from build123d import *

# Parameters (mm, degrees)
CHAMFER_1_SIZE           = 1
SKETCH_4_W               = 2
SKETCH_4_H               = 1
CUT_EXTRUDE_1_DEPTH      = 35.092374778
CUT_EXTRUDE_2_REACH      = 36.092
PATTERN_CIRCULAR_3_COUNT = 18
SKETCH_7_R               = 25
CUT_EXTRUDE_3_DEPTH      = 21
SKETCH_8_R               = 5
EXTRUDE_1_DEPTH          = 7
SKETCH_10_R              = 3
CUT_EXTRUDE_4_DEPTH      = 10
SKETCH_11_R              = 1.525
CUT_EXTRUDE_5_DEPTH      = 46


with BuildPart() as part:
    # 草图1 → 旋转1 (revolve)
    with BuildSketch(Plane.XY, mode=Mode.PRIVATE) as revolve_1_sk:
        Polygon((0, 2.7506), (0, 13.753), (28, 13.753), (28, 5.5012), (20, 5.5012), (20, 2.7506), align=None)
    revolve(revolve_1_sk.sketch.rotate(Axis((0, 0, 0), (1, 0, 0)), 90), axis=Axis((0, 0, 0), (1, 0, 0)))

    # 倒角1
    chamfer_1_edges = [part.edges().sort_by_distance(p)[0] for p in [
        (20, 0, -2.7506),
        (0, 0, -2.7506),
    ]]
    chamfer(chamfer_1_edges, length=CHAMFER_1_SIZE)

    # 草图4 → 切除-拉伸1 (cut, through all)
    with BuildSketch(Plane.ZY):
        with Locations((0, 3.062381775)):
            Rectangle(SKETCH_4_W, SKETCH_4_H)
    extrude(amount=-CUT_EXTRUDE_1_DEPTH, mode=Mode.SUBTRACT)

    # 草图6 → 切除-拉伸2 (cut, up to next)
    with BuildSketch(Plane(origin=(0, 0, 0), x_dir=(0, 0, -1), z_dir=(1, 0, 0)), mode=Mode.PRIVATE) as cut_extrude_2_sk1:
        with BuildLine():
            Line((1.574067282, 13.17215513), (1.548371997, 12.962883824))
            ThreePointArc((1.548371997, 12.962883824), (0, 11.593), (-1.548371997, 12.962883824))
            Line((-1.548371997, 12.962883824), (-1.574067282, 13.17215513))
            ThreePointArc((-1.574067282, 13.17215513), (-1.761240253, 13.496717776), (-2.124642597, 13.587895453))
            ThreePointArc((-2.124642597, 13.587895453), (-2.36143787, 13.548749765), (-2.597513963, 13.505477785))
            Line((-2.597513963, 13.505477785), (-2.794161951, 15.107047128))
            ThreePointArc((-2.794161951, 15.107047128), (0, 15.363274844), (2.794161951, 15.107047128))
            Line((2.794161951, 15.107047128), (2.597513963, 13.505477785))
            ThreePointArc((2.597513963, 13.505477785), (2.36143787, 13.548749765), (2.124642597, 13.587895453))
            ThreePointArc((2.124642597, 13.587895453), (1.761240253, 13.496717776), (1.574067282, 13.17215513))
        make_face()
    cut_extrude_2_tool1 = extrude(cut_extrude_2_sk1.sketch, amount=CUT_EXTRUDE_2_REACH, mode=Mode.PRIVATE) & part.part
    cut_extrude_2 = cut_extrude_2_tool1.solids().sort_by_distance((0, 13.819423, 0))[0]
    add(cut_extrude_2, mode=Mode.SUBTRACT)

    # 阵列(圆周)3: 切除-拉伸2 ×18 about axis
    pattern_circular_3_axis = Axis((0, 0, 0), (1, 0, 0))
    for i in range(1, PATTERN_CIRCULAR_3_COUNT):
        add(cut_extrude_2.rotate(pattern_circular_3_axis, i * 360 / PATTERN_CIRCULAR_3_COUNT), mode=Mode.SUBTRACT)

    # 草图7 → 切除-拉伸3 (cut)
    with BuildSketch(Plane(origin=(28, 0, 0), x_dir=(0, 0, -1), z_dir=(1, 0, 0))):
        Circle(SKETCH_7_R)
    extrude(amount=-CUT_EXTRUDE_3_DEPTH, mode=Mode.SUBTRACT)

    # 草图8 → 凸台-拉伸1 (add)
    with BuildSketch(Plane(origin=(7, 0, 0), x_dir=(0, 0, -1), z_dir=(1, 0, 0))):
        Circle(SKETCH_8_R)
    extrude(amount=-EXTRUDE_1_DEPTH)

    # 草图10 → 切除-拉伸4 (cut)
    with BuildSketch(Plane(origin=(7, 0, 0), x_dir=(0, 0, -1), z_dir=(1, 0, 0))):
        Circle(SKETCH_10_R)
    extrude(amount=-CUT_EXTRUDE_4_DEPTH, mode=Mode.SUBTRACT)

    # 草图11 → 切除-拉伸5 (cut)
    with BuildSketch(Plane(origin=(7, 0, 0), x_dir=(0, 0, -1), z_dir=(1, 0, 0))):
        with Locations((0, 7.5)):
            Circle(SKETCH_11_R)
        with Locations((7.5, 0)):
            Circle(SKETCH_11_R)
        with Locations((0, -7.5)):
            Circle(SKETCH_11_R)
        with Locations((-7.5, 0)):
            Circle(SKETCH_11_R)
    extrude(amount=-CUT_EXTRUDE_5_DEPTH, mode=Mode.SUBTRACT)


solid = part.part
Model file for the job. Use its own axes, mm. Round coordinates to 2 decimals unless told otherwise and drop trailing zeros. Order: outer loops, then holes, each group sorted by start corner. A loop starts at its lowest first (then second) coordinate and runs counter-clockwise, first axis right, second up. Notation, with made-up numbers: M -0.75,83 L 12.25,83 A6 ccw 12.25,88 Z; hole C 62,-39.75 d2. An arc over 180 degrees is marked long. Write each question's results on one line, items separated by ' | '. Start each with the question number.
(1) Saw through at C-C, the plane x = 6. State how many separate pieces and enclosed holes the cut face has, then the cut area to 3 significant figures.
(2) Saw through at A-A, the plane z = 0. Give the cut face in (x, y) (3 decimals), then the cut area to 3 significant figures.
(3) Probe probe 1 along Y at (x, z) = (5, 0) (3 decimals); probe 2 along Y at (x, z) = (4.5, 12.5); probe 3 along Z at (x, y) = (5, -1.25). List the from-to ranges inside material, lowest first. Write a range as from..to.
(4) Saw through at D-D, the plane y = -9.75. Give the cut face in (x, z).
(5) Saw through at B-B, the plane y = 7.5. Give the cut face in (x, z) (3 decimals), then the cut area to 3 significant figures.
(6) Drop flat-ended pins along their axis: pin 1 (8 mm diameter, centred on y = 0, z = 0, fed in from -X); pin 2 (1.5 mm diameter, centred on x = 5.5, y = 3.5, fed in from -Z); pin 3 (4 mm diameter, centred on x = 5.5, y = -8, fed in from +Z); pin 4 (2 mm diameter, centred on x = 1, y = 3.5, fed in from +Z). Give the stop position or say it passes through.
(7) Two-plate mould, pull along Y, no slides. Class faces 1 (the face through (7, 0.2, 3.2)), 2 (the face through (3.451, -11.593, 0.032)), 3 (the face through (3.451, 2.044, 11.412)): pulls with the +Y half, pulls with the -Y half, needs draft (parallel to the pull), parting line crosses it, or undercut.
Established:
1) separate pieces: 1 | enclosed holes: 5 | area: 433 mm^2
2) outline: M 0,-11.593 L 7,-11.593 L 7,-9.025 L 0,-9.025 Z; M 0,-5.975 L 7,-5.975 L 7,-3 L 0,-3 Z; M 0,3 L 7,3 L 7,5.975 L 0,5.975 Z; M 0,9.025 L 7,9.025 L 7,11.593 L 0,11.593 Z | area: 77.6 mm^2
3) probe 1: y = -11.593..-9.025, -5.975..-3, 3..5.975, 9.025..11.593 | probe 2: y = -5.25..-3.78, -0.79..0.79, 3.78..5.25 | probe 3: z = -11.79..-8.37, -6.63..-2.73, 2.73..6.63, 8.37..11.79
4) outline: M 0,-6.93 L 7,-6.93 L 7,6.93 L 0,6.93 Z
5) outline: M 0,-10.134 L 7,-10.134 L 7,-1.525 L 0,-1.525 Z; M 0,1.525 L 7,1.525 L 7,10.134 L 0,10.134 Z | area: 121 mm^2
6) pin 1: stops at x = 0 | pin 2: stops at z = -13.04 | pin 3: stops at z = 10.81 | pin 4: stops at z = 13.04
7) face 1: needs draft | face 2: pulls with the -Y half | face 3: undercut
